Could you check a few things on this model? Use its own coordinates, in mm. A direction names the side the tool comes from. Round coordinates to 2 decimals unless told otherwise and drop trailing zeros. Write each loop counter-clockwise with the first axis right and the second up, starting at its lowest first coordinate (ties: lowest second). Pieces come first, ordered by that corner, then holes. Notation, with made-up numbers: (43.5, 38) -> (100.5, 38) arc R26 ccw to (100.5, 54) -> close; hole circle Ø1 at (-14, -7). An arc over 180 degrees is marked (long way). Answer in a Markdown table with one row per item. Add a question column.
```python
from build123d import *

# Parameters (mm, degrees)
CROQUIS1_W              = 51
CROQUIS1_H              = 102
SALIENTE_EXTRUIR1_DEPTH = 30
VACIADO1_T              = 3
CROQUIS5_R              = 1.5
SALIENTE_EXTRUIR2_DEPTH = 5
CROQUIS8_R              = 3
SALIENTE_EXTRUIR3_DEPTH = 30
CROQUIS10_R             = 1.5
CORTAR_EXTRUIR1_DEPTH   = 25
CROQUIS14_W             = 25
CROQUIS14_H             = 7
CORTAR_EXTRUIR3_DEPTH   = 3
CROQUIS15_W             = 8.5
CROQUIS15_H             = 4.8
CORTAR_EXTRUIR4_DEPTH   = 3
CROQUIS16_W             = 7.48
CROQUIS16_H             = 6
CORTAR_EXTRUIR5_DEPTH   = 3
CROQUIS17_R             = 2.5
CORTAR_EXTRUIR6_DEPTH   = 3
CROQUIS18_W             = 15
CROQUIS18_H             = 9
CORTAR_EXTRUIR7_DEPTH   = 54


with BuildPart() as part:
    # Croquis1 → Saliente-Extruir1 (new body)
    with BuildSketch(Plane(origin=(0, 0, 0), x_dir=(1, 0, 0), z_dir=(0, 1, 0))):
        Rectangle(CROQUIS1_W, CROQUIS1_H)
    extrude(amount=SALIENTE_EXTRUIR1_DEPTH)

    # Vaciado1
    vaciado1_openings = [part.faces().sort_by_distance(p)[0] for p in [
        (0, 30, 0),
    ]]
    offset(amount=VACIADO1_T, openings=vaciado1_openings, kind=Kind.INTERSECTION)

    # Croquis5 → Saliente-Extruir2 (add)
    # profile 1 of 4: a face of its own
    with BuildSketch(Plane.XZ.offset(3)):
        with BuildLine():
            Line((28.5, 54), (35.5, 54))
            ThreePointArc((35.5, 54), (38.999999038, 50.49999936), (35.49999872, 47))
            Line((35.49999872, 47), (28.5, 47))
            Line((28.5, 47), (28.5, 54))
        make_face()
        with Locations(Location((35.499999038, 50.5, 0), (0, 0, 270))):
            Circle(CROQUIS5_R, mode=Mode.SUBTRACT)
    # profile 2 of 4: a face of its own
    with BuildSketch(Plane.XZ.offset(3)):
        with BuildLine():
            Line((-28.5, 54), (-35.5, 54))
            ThreePointArc((-35.5, 54), (-38.999999054, 50.499999378), (-35.499998756, 47))
            Line((-35.499998756, 47), (-28.5, 47))
            Line((-28.5, 47), (-28.5, 54))
        make_face()
        with Locations(Location((-35.499999054, 50.5, 0), (0, 0, 270))):
            Circle(CROQUIS5_R, mode=Mode.SUBTRACT)
    # profile 3 of 4: a face of its own
    with BuildSketch(Plane.XZ.offset(3)):
        with BuildLine():
            Line((-28.5, -54), (-35.5, -54))
            ThreePointArc((-35.5, -54), (-38.999999038, -50.49999936), (-35.49999872, -47))
            Line((-35.49999872, -47), (-28.5, -47))
            Line((-28.5, -47), (-28.5, -54))
        make_face()
        with Locations(Location((-35.499999038, -50.5, 0), (0, 0, 270))):
            Circle(CROQUIS5_R, mode=Mode.SUBTRACT)
    # profile 4 of 4: a face of its own
    with BuildSketch(Plane.XZ.offset(3)):
        with BuildLine():
            Line((28.5, -54), (35.5, -54))
            ThreePointArc((35.5, -54), (38.999999041, -50.499999359), (35.499998718, -47))
            Line((35.499998718, -47), (28.5, -47))
            Line((28.5, -47), (28.5, -54))
        make_face()
        with Locations(Location((35.499999041, -50.5, 0), (0, 0, 270))):
            Circle(CROQUIS5_R, mode=Mode.SUBTRACT)
    extrude(amount=-SALIENTE_EXTRUIR2_DEPTH)

    # Croquis8 → Saliente-Extruir3 (add)
    with BuildSketch(Plane(origin=(0, 0, 0), x_dir=(1, 0, 0), z_dir=(0, 1, 0))):
        with Locations((-25.5, 51)):
            Circle(CROQUIS8_R)
        with Locations((25.5, 51)):
            Circle(CROQUIS8_R)
        with Locations((25.5, -51)):
            Circle(CROQUIS8_R)
        with Locations((-25.5, -51)):
            Circle(CROQUIS8_R)
    extrude(amount=SALIENTE_EXTRUIR3_DEPTH)

    # Croquis10 → Cortar-Extruir1 (cut)
    with BuildSketch(Plane(origin=(0, 30, 0), x_dir=(1, 0, 0), z_dir=(0, 1, 0))):
        with Locations(Location((-25.5, 51, 0), (0, 0, 270))):
            Circle(CROQUIS10_R)
        with Locations(Location((25.5, 51, 0), (0, 0, 270))):
            Circle(CROQUIS10_R)
        with Locations(Location((-25.5, -51, 0), (0, 0, 270))):
            Circle(CROQUIS10_R)
        with Locations(Location((25.5, -51, 0), (0, 0, 270))):
            Circle(CROQUIS10_R)
    extrude(amount=-CORTAR_EXTRUIR1_DEPTH, mode=Mode.SUBTRACT)

    # Croquis14 → Cortar-Extruir3 (cut)
    with BuildSketch(Plane(origin=(28.5, 0, 0), x_dir=(0, 0, -1), z_dir=(1, 0, 0))):
        with Locations((-32.5, 26.5)):
            Rectangle(CROQUIS14_W, CROQUIS14_H)
    extrude(amount=-CORTAR_EXTRUIR3_DEPTH, mode=Mode.SUBTRACT)

    # Croquis15 → Cortar-Extruir4 (cut)
    with BuildSketch(Plane.ZY.offset(28.5)):
        with Locations((-37.75, 22.6)):
            Rectangle(CROQUIS15_W, CROQUIS15_H)
    extrude(amount=-CORTAR_EXTRUIR4_DEPTH, mode=Mode.SUBTRACT)

    # Croquis16 → Cortar-Extruir5 (cut)
    with BuildSketch(Plane(origin=(28.5, 0, 0), x_dir=(0, 0, -1), z_dir=(1, 0, 0))):
        with Locations((38.02, 22)):
            Rectangle(CROQUIS16_W, CROQUIS16_H)
    extrude(amount=-CORTAR_EXTRUIR5_DEPTH, mode=Mode.SUBTRACT)

    # Croquis17 → Cortar-Extruir6 (cut)
    with BuildSketch(Plane.XZ.offset(3)):
        with Locations(Location((0, -42, 0), (0, 0, 270))):
            Circle(CROQUIS17_R)
    extrude(amount=-CORTAR_EXTRUIR6_DEPTH, mode=Mode.SUBTRACT)

    # Croquis18 → Cortar-Extruir7 (cut)
    with BuildSketch(Plane(origin=(0, 0, -54), x_dir=(-1, 0, 0), z_dir=(0, 0, -1))):
        with Locations((0, 20.5)):
            Rectangle(CROQUIS18_W, CROQUIS18_H)
    extrude(amount=-CORTAR_EXTRUIR7_DEPTH, mode=Mode.SUBTRACT)


solid = part.part
```
(1) Suppose I cut it at C-C, the plane x = -9.5. Please give me the cut outline in (y, z).
(2) For P1, Ø1, axis at x = -6.5, z = -5, coming from the +Y side; P2, Ø10, axis at y = 12.5, z = 14, coming from the -X side; P3, Ø5, axis at y = 4.5, z = -22.5, coming from the +X side, each with a flat end and sliding along its axis, tell me the tip position at first contact or that it passes through.
(3) Suppose I cut it at A-A, the plane y = 9. Please give me the cut outline in (x, z), then the cut area to 3 significant figures.
(4) I need wall thicknesses on L1, parallel to X at y = -0.05, z = -50.5; L2, parallel to X at y = 0.95, z = -50.5; L3, parallel to Z at x = -25, y = 12. Which ranges of each line are inside material? Lowest first, please.
(5) Suppose I cut it at B-B, the plane z = 34. Please give me the cut outline in (x, y).
(6) If we mould it in two halves opening along Z, with no side actions, what happens to faces 1 (the face through (-33.7, 2, -50.5)), 2 (the face through (0, 13, 54)), 3 (the face through (-27, 20.2, -38))? For each: pulls with the +Z half, pulls with the -Z half, needs draft (parallel to the pull), parting line crosses it, or undercut.
(7) On a 3-axis mill with a long thin cutter (end or side, diameter ignored), from which of +Z, -Z, +X, -X, +Y, -Y can I reach the whole of each face in a straight line? I mean faces 4 (the face through (-24.49, 17.68, 49.89)), 5 (the face through (27, 22, -41.76)), 6 (the face through (27, 26, 20)), 7 (the face through (0, 16, -53)). Say none if no direction works.
Response:
| question | item | result |
|---|---|---|
| 1 | outline | (-3, -54) -> (30, -54) -> (30, -51) -> (0, -51) -> (0, 51) -> (30, 51) -> (30, 54) -> (-3, 54) -> close |
| 2 | P1 | y = 0 |
| 2 | P2 | x = -28.5 |
| 2 | P3 | x = 28.5 |
| 3 | outline | (-28.5, -54) -> (28.5, -54) -> (28.5, 54) -> (-28.5, 54) -> close; hole circle Ø3 at (-25.5, -51); hole circle Ø3 at (-25.5, 51); hole (-25.5, -48) arc R3 cw to (-22.5, -51) -> (22.5, -51) arc R3 cw to (25.5, -48) -> (25.5, 48) arc R3 cw to (22.5, 51) -> (-22.5, 51) arc R3 cw to (-25.5, 48) -> close; hole circle Ø3 at (25.5, -51); hole circle Ø3 at (25.5, 51) |
| 3 | area | 954 mm² |
| 4 | L1 | -39 to -37, -34 to 34, 37 to 39 |
| 4 | L2 | -39 to -37, -34 to -22.54, 22.54 to 34, 37 to 39 |
| 4 | L3 | -54 to -52.41, -49.59 to -48.04, 48.04 to 49.59, 52.41 to 54 |
| 5 | outline | (-28.5, -3) -> (28.5, -3) -> (28.5, 23) -> (25.5, 23) -> (25.5, 0) -> (-25.5, 0) -> (-25.5, 30) -> (-28.5, 30) -> close |
| 6 | face 1 | needs draft |
| 6 | face 2 | pulls with the +Z half |
| 6 | face 3 | undercut |
| 7 | face 4 | +Y |
| 7 | face 5 | +X |
| 7 | face 6 | +X, +Y |
| 7 | face 7 | -Z |
